Autodesk Inventor part; units mm, degrees
ref_plane "YZ Plane" through (0, 0, 0) normal (1, 0, 0) x (0, 1, 0)
ref_plane "XZ Plane" through (0, 0, 0) normal (0, 1, 0) x (-1, 0, 0)
ref_plane "XY Plane" through (0, 0, 0) normal (0, 0, 1) x (1, 0, 0)
sketch "Sketch4" plane through (0, 0, 0) normal (0, 1, 0) x (-1, 0, 0)
  line L0 (-19.05, 6.35) -> (2.3114, 6.35)
  line L1 (19.05, 6.35) -> (19.05, -6.35)
  line L2 (19.05, -6.35) -> (10.3886, -6.35)
  line L3 (-19.05, -6.35) -> (-19.05, 6.35)
  line L4 (-19.05, 6.35) -> (19.05, -6.35) construction
  line L5 (19.05, 6.35) -> (-19.05, -6.35) construction
  line L6 (-2.3114, 2.3114) -> (2.3114, 2.3114)
  line L7 (2.3114, 2.3114) -> (2.3114, -2.3114)
  line L8 (2.3114, -2.3114) -> (-2.3114, -2.3114)
  line L9 (-2.3114, -2.3114) -> (-2.3114, 2.3114)
  line L10 (-2.3114, 2.3114) -> (2.3114, -2.3114) construction
  line L11 (2.3114, 2.3114) -> (-2.3114, -2.3114) construction
  line L12 (10.3886, 2.3114) -> (15.0114, 2.3114)
  line L13 (15.0114, 2.3114) -> (15.0114, -2.3114)
  line L14 (15.0114, -2.3114) -> (10.3886, -2.3114)
  line L15 (10.3886, -2.3114) -> (10.3886, 2.3114)
  line L16 (10.3886, 2.3114) -> (15.0114, -2.3114) construction
  line L17 (15.0114, 2.3114) -> (10.3886, -2.3114) construction
  line L18 (10.3886, 6.35) -> (10.3886, 7.62)
  line L19 (2.3114, 6.35) -> (2.3114, 7.62)
  line L20 (2.3114, 7.62) -> (10.3886, 7.62)
  line L21 (10.3886, -6.35) -> (10.3886, -7.62)
  line L22 (2.3114, -6.35) -> (2.3114, -7.62)
  line L23 (2.3114, -7.62) -> (10.3886, -7.62)
  line L24 (10.3886, 6.35) -> (19.05, 6.35)
  line L25 (2.3114, -6.35) -> (-19.05, -6.35)
  point P0 (0, 0)
  point P1 (12.7, 0)
  dimension "d14" = 38.1
  dimension "d15" = 12.7
  dimension "d16" = 4.6228
  dimension "d17" = 4.6228
  dimension "d18" = 4.6228
  dimension "d19" = 12.7
  dimension "d20" = 1.27
  dimension "d27" = 1.27
extrude "Extrusion2" add sketch "Sketch4" along normal blind 1.1684
sketch "Sketch5" plane through (0, 1.1684, 0) normal (0, 1, 0) x (1, 0, 0)
  circle A0 centre (-6.35, -4.0005) radius 2.3876
  point P0 (0, 0)
  point P1 (-6.35, 0)
  dimension "d24" = 6.35
  dimension "d25" = 4.7752
  dimension "d26" = 4.0005
sketch "Sketch6" plane through (0, 1.1684, 0) normal (0, 1, 0) x (1, 0, 0)
  circle A0 centre (-6.35, 4.0132) radius 2.3876
  point P0 (0, 0)
  point P1 (-6.35, 0)
  dimension "d29" = 6.35
  dimension "d30" = 4.7752
  dimension "d31" = 4.0132
extrude "Extrusion3" add sketch "Sketch5" along normal blind 8.001
extrude "Extrusion4" add sketch "Sketch6" along normal blind 8.001
sketch "Sketch8" plane through (0, 1.1684, 0) normal (0, 1, 0) x (1, 0, 0)
  circle A0 centre (12.7, 0) radius 4.0005
  point P0 (0, 0)
  dimension "d41" = 12.7
  dimension "d45" = 8.001
extrude "Extrusion6" add sketch "Sketch8" along normal blind 6.8326
sketch "Sketch9" plane through (12.7, 8.001, 0) normal (0, 1, 0) x (1, 0, 0)
  circle A0 centre (0, 0) radius 2.8067
  point P0 (-12.7, 0)
  dimension "d48" = 5.6134
extrude "Extrusion7" cut sketch "Sketch9" against normal blind 0.7874
sketch "Sketch10" plane through (12.7, 7.2136, 0) normal (0, 1, 0) x (1, 0, 0)
  circle A0 centre (0, 0) radius 2.4003
  point P0 (-12.7, 0)
  dimension "d51" = 4.8006
extrude "Extrusion8" cut sketch "Sketch10" against normal through all
sketch "Sketch11" plane through (0, 0, 0) normal (0, -1, 0) x (1, 0, 0)
  circle A0 centre (12.7, 0) radius 4.0005
  circle A1 centre (12.7, 0) radius 2.8067
  point P0 (0, 0)
  dimension "d54" = 12.7
  dimension "d55" = 5.6134
extrude "Extrusion9" cut sketch "Sketch11" against normal blind 0.7874 contours A1
properties part number "VexLegoWidget2"
Could you check a few things on this model? Use its own coordinates, in mm. A direction names the side the tool comes from. Coordinates: 2 decimals unless noted, no trailing zeros. Order: outer loops, then holes, each group sorted by start corner. A loop starts at its lowest first (then second) coordinate and runs counter-clockwise, first axis right, second up. Notation, with made-up numbers: (-11, -1) - (43, -1) arc R23 cw to (43, 38) - close; hole circle Ø10 at (3.5, 56). An arc over 180 degrees is marked (long way). Answer in a Markdown table with one row per item. Add a question column.
(1) I need wall thicknesses on L1, parallel to Z at x = 12.7, y = 7.8; L2, parallel to X at y = 5.5, z = -2; L3, parallel to X at y = 1, z = 1. Which ranges of each line are inside material? Lowest first, please.
(2) On a 3-axis mill with a long thin cutter (end or side, diameter ignored), from which of +Z, -Z, +X, -X, +Y, -Y can I reach the whole of each face in a straight line? I mean faces 5 (the face through (-5.25, 5.11, 1.88)), 6 (the face through (2.311, 1, 0)), 7 (the face through (-2.311, 1, 7)), 8 (the face through (9.896, 0.388, 0.123)), 9 (the face through (-15, 1, 6.35)). Say none if no direction works.
(3) Will these pins go through, and if not, where does the flat tip stop? pin 1 (2 mm diameter, centred on x = -11.5, z = 1.5, fed in from +Y); pin 2 (1.3 mm diameter, centred on x = -1, y = 0.5, fed in from -Z); pin 3 (3 mm diameter, centred on x = 13, z = 2.5, fed in from +Y).
(4) If we section it at D-D, the plane y = 5.5: Please give me the cut outline in (x, z), then the cut area to 3 significant figures.
(5) If we mould it in two halves opening along X, with no side actions, what happens to faces 1 (the face through (11, 7.214, -2)), 2 (the face through (0, 0, 3)), 3 (the face through (-10.389, 1, -7)), 4 (the face through (11, 0.787, 2))? For each: released by +X, released by -X, zero draft, split by the parting line, or undercut.
(6) If we section it at C-C, the plane x = -6.35: Please give me the cut outline in (y, z), then the cut area to 3 significant figures.
(7) If we section it at A-A, the plane x = -1.5: Please give me the cut outline in (y, z), then the cut area to 3 significant figures.
(8) If we section it at B-B, the plane z = 0: Please give me the cut outline in (x, y).
Results are:
| question | item | result |
|---|---|---|
| 1 | L1 | z = -4 to -2.81, 2.81 to 4 |
| 1 | L2 | x = -7.63 to -5.07, 9.24 to 11.37, 14.03 to 16.16 |
| 1 | L3 | x = -19.05 to -15.01, -10.39 to -2.31, 2.31 to 10.52, 14.88 to 19.05 |
| 2 | face 5 | +Y |
| 2 | face 6 | +Y, -Y |
| 2 | face 7 | +Z, +X, +Y, -Y |
| 2 | face 8 | -Y |
| 2 | face 9 | +Z, -X, +Y, -Y |
| 3 | pin 1 | stops at y = 1.17 |
| 3 | pin 2 | stops at z = -6.35 |
| 3 | pin 3 | stops at y = 8 |
| 4 | outline | circle Ø4.78 at (-6.35, -4.01); circle Ø4.78 at (-6.35, 4); circle Ø8 at (12.7, 0); hole circle Ø4.8 at (12.7, 0) |
| 4 | area | 68.0 mm2 |
| 5 | face 1 | undercut |
| 5 | face 2 | zero draft |
| 5 | face 3 | released by -X |
| 5 | face 4 | undercut |
| 6 | outline | (0, -7.62) - (1.17, -7.62) - (1.17, -6.4) - (9.17, -6.4) - (9.17, -1.63) - (1.17, -1.63) - (1.17, 1.61) - (9.17, 1.61) - (9.17, 6.39) - (1.17, 6.39) - (1.17, 7.62) - (0, 7.62) - close |
| 6 | area | 94.2 mm2 |
| 7 | outline | (0, -6.35) - (1.17, -6.35) - (1.17, -2.31) - (0, -2.31) - close; (0, 2.31) - (1.17, 2.31) - (1.17, 6.35) - (0, 6.35) - close |
| 7 | area | 9.44 mm2 |
| 8 | outline | (-19.05, 0) - (-15.01, 0) - (-15.01, 1.17) - (-19.05, 1.17) - close; (-10.39, 0) - (-2.31, 0) - (-2.31, 1.17) - (-10.39, 1.17) - close; (2.31, 0) - (9.89, 0) - (9.89, 0.79) - (10.3, 0.79) - (10.3, 7.21) - (9.89, 7.21) - (9.89, 8) - (8.7, 8) - (8.7, 1.17) - (2.31, 1.17) - close; (15.1, 0.79) - (15.51, 0.79) - (15.51, 0) - (19.05, 0) - (19.05, 1.17) - (16.7, 1.17) - (16.7, 8) - (15.51, 8) - (15.51, 7.21) - (15.1, 7.21) - close |
